from build123d import *

# Parameters (mm, degrees)
F0_R     = 29
F1_DEPTH = 30
F3_R     = 27
F4_DEPTH = 27
F5_R     = 3
F6_R     = 3


with BuildPart() as f1:
    # F0 (on Top) → F1 (new body)
    with BuildSketch(Plane.XY):
        Circle(F0_R)
    extrude(amount=F1_DEPTH)

    # F3 (on offset) → F4 (cut)
    with BuildSketch(Plane.XY.offset(30)):
        Circle(F3_R)
    extrude(amount=-F4_DEPTH, mode=Mode.SUBTRACT)

    # F5
    f5_edges = [f1.edges().sort_by_distance(p)[0] for p in [
        (-27, 0, 3),
    ]]
    fillet(f5_edges, radius=F5_R)

    # F6
    f6_edges = [f1.edges().sort_by_distance(p)[0] for p in [
        (-29, 0, 0),
    ]]
    fillet(f6_edges, radius=F6_R)

    # F7 (on Right) → F8 (revolve)
    with BuildSketch(Plane.YZ):
        Polygon((-3, 3), (0, 3), (0, 38), align=None)
    revolve(axis=Axis((0, 0, 20.5), (0, 0, 1)))


solid = f1.part
Read the model definition and answer for the solid it produces. Units are mm, in the model's axes. A direction names the side the tool comes from. Coordinates: 2 decimals unless noted, no trailing zeros. Loops run counter-clockwise (first coordinate to the right, second up) from the corner with the lowest first, then second, coordinate; pieces in that order, holes last. Notation, with made-up numbers: (82.25, 56) -> (111.25, 56) arc R8 ccw to (111.25, 70) -> close; hole circle Ø7 at (56, -30.75). An arc over 180 degrees is marked (long way). Write item = value, one per line. Start each with the question number.
1) Find the intervals of material crossed by L1, parallel to Y at x = 0, z = 20.5; L2, parallel to Y at x = 0, z = 27; L3, parallel to Y at x = -10, z = 10, in increasing order. Write a range as from..to.
2) For faces 1 (the face through (0, 0, 0)), 2 (the face through (5, 0, 3)), determine the directions among +Z, -Z, +X, -X, +Y, -Y from which every point of the face is accessible in a straight line to the end or side of a thin tool.
3) Given P1, Ø5, axis at y = -11, z = 13, coming from the +X side; P2, Ø2, axis at x = -15, z = 14.5, coming from the +Y side; P3, Ø4, axis at x = -20.5, y = 1.5, coming from the +Z side; P4, Ø2, axis at x = -14, y = -8, coming from the -Z side, each flat-ended and moving along its own axis, determine where each tip first touches the part or whether it passes through.
4) The mould has two halves that part along X. Classify faces 3 (the face through (13.38, -25.73, 16.31)), 4 (the face through (-1.485, 0.33, 20.255)), 5 (the face through (8, -26, 30)), 6 (the face through (-5.85, -26.36, 18.17)): pulls with the +X half, pulls with the -X half, needs draft (parallel to the pull), parting line crosses it, or undercut.
5) The part is cut by section A-A, the plane z = 10.5. Determine the outline of the cut face in (x, y), plus the area to 3 significant figures.
Result:
q1.L1 = -29..-27, -1.5..1.5, 27..29
q1.L2 = -29..-27, -0.94..0.94, 27..29
q1.L3 = -27.22..-25.08, 25.08..27.22
q2.face_1 = -Z, +X, -X, +Y, -Y
q2.face_2 = +Z
q3.P1 = 27.73
q3.P2 = 25.4
q3.P3 = 3
q3.P4 = 0
q4.face_3 = parting line crosses it
q4.face_4 = undercut
q4.face_5 = needs draft
q4.face_6 = undercut
q5.outline = circle Ø58 at (0, 0); circle Ø4.71 at (0, 0); hole circle Ø54 at (0, 0)
q5.area = 369 mm²
